Part model, mm, in its own coordinate system. Give positions to 0.01 mm unless a question says otherwise; leave off trailing zeros. Write each loop counter-clockwise with the first axis right and the second up, starting at its lowest first coordinate (ties: lowest second). Pieces come first, ordered by that corner, then holes. Notation, with made-up numbers: (42, -5.5) - (46, -5.5) arc R11 cw to (46, 7.5) - close; hole circle Ø5 at (-26.5, 58.5). An arc over 180 degrees is marked (long way). Answer in a Markdown table with one row per item. Add a question column.
1. Probe line 1 along X through (y, z) = (-2.5, -51.05); line 2 along Y through (x, z) = (-9.5, -51.05); line 3 along X through (y, z) = (1, -51.1). List the from-to ranges inside material, lowest first.
2. Band-saw the part on B-B on y = 9. Write the cut outline in (x, z), plus the area to 3 significant figures.
3. Band-saw the part on D-D on y = -2. Write the cut outline in (x, z), plus the area to 3 significant figures.
4. Band-saw the part on A-A on x = -17. Write the cut outline in (y, z).
5. Band-saw the part on C-C on x = -8.5. Write the cut outline in (y, z).
```python
from build123d import *

# Parameters (mm, degrees)
EXTRUDE_START       = -3.8
SKETCH_1_R          = 25.801076528
SKETCH_1_R_2        = 1.549997321
SKETCH_1_R_3        = 1.54999944
EXTRUDE_1_DEPTH     = 0.2
CUT_EXTRUDE_START   = -3.8
SKETCH_2_W          = 3.794
SKETCH_2_H          = 3.794
SKETCH_2_W_2        = 4.175
SKETCH_2_H_2        = 4.556
SKETCH_2_W_3        = 4.048
SKETCH_2_H_3        = 4.683
CUT_EXTRUDE_1_DEPTH = 0.2
CUT_EXTRUDE_2_DEPTH = 0.2
CUT_EXTRUDE_3_DEPTH = 0.2
CUT_EXTRUDE_4_DEPTH = 0.2
CUT_EXTRUDE_5_DEPTH = 0.2


with BuildPart() as part:
    # 草图1 → 凸台-拉伸1 (new body)
    with BuildSketch(Plane(origin=(0, 0, -54.8040151), x_dir=(-1, 0, 0), z_dir=(0, 0, -1)).offset(EXTRUDE_START)):
        with Locations(Location((24.698490112, -1.512152456, 0), (0, 0, 180))):
            Circle(SKETCH_1_R)
        with Locations(Location((24.698490112, 21.537847164, 0), (0, 0, 180))):
            Circle(SKETCH_1_R_2, mode=Mode.SUBTRACT)
        with Locations(Location((24.698490112, -24.562152076, 0), (0, 0, 180))):
            Circle(SKETCH_1_R_3, mode=Mode.SUBTRACT)
    extrude(amount=EXTRUDE_1_DEPTH)

    # 草图2 → 切除-拉伸1 (cut)
    with BuildSketch(Plane(origin=(0, 0, -54.8040151), x_dir=(-1, 0, 0), z_dir=(0, 0, -1)).offset(CUT_EXTRUDE_START)):
        with Locations((23.362494109, -1.270150744)):
            Rectangle(SKETCH_2_W, SKETCH_2_H)
        with Locations((34.093992827, 9.14385072)):
            Rectangle(SKETCH_2_W_2, SKETCH_2_H_2)
        with Locations((41.967993376, 9.397848523)):
            Rectangle(SKETCH_2_W_2, SKETCH_2_H_2)
        with Locations((34.157492278, -11.874650561)):
            Rectangle(SKETCH_2_W_3, SKETCH_2_H_3)
        with Locations((42.031492827, -11.874650561)):
            Rectangle(SKETCH_2_W_3, SKETCH_2_H_3)
    extrude(amount=CUT_EXTRUDE_1_DEPTH, mode=Mode.SUBTRACT)

    # 草图3 → 切除-拉伸2 (cut)
    with BuildSketch(Plane(origin=(0, 0, -54.8040151), x_dir=(-1, 0, 0), z_dir=(0, 0, -1)).offset(CUT_EXTRUDE_START)):
        Polygon((15.882224059, 13.556279819), (9.63139829, 7.305454051), (2.996403479, 13.940448863), (9.247230868, 20.191276253), align=None)
    extrude(amount=CUT_EXTRUDE_2_DEPTH, mode=Mode.SUBTRACT)

    # 草图4 → 切除-拉伸3 (cut)
    with BuildSketch(Plane(origin=(0, 0, -54.8040151), x_dir=(-1, 0, 0), z_dir=(0, 0, -1)).offset(CUT_EXTRUDE_START)):
        Polygon((7.030438471, 4.406785556), (7.030438471, 6.006785556), (10.230438471, 6.006785556), (10.230438471, 4.406785556), (8.630438471, 4.406785556), align=None)
        Polygon((7.030438471, 0.086785556), (7.030438471, 1.686785556), (10.230438471, 1.686785556), (10.230438471, 0.086785556), (8.630438471, 0.086785556), align=None)
        Polygon((7.030438471, -4.363214444), (7.030438471, -2.763214444), (10.230438471, -2.763214444), (10.230438471, -4.363214444), (8.630438471, -4.363214444), align=None)
        Polygon((7.030438471, -9.573214444), (7.030438471, -7.973214444), (10.230438471, -7.973214444), (10.230438471, -9.573214444), (8.630438471, -9.573214444), align=None)
    extrude(amount=CUT_EXTRUDE_3_DEPTH, mode=Mode.SUBTRACT)

    # 草图5 → 切除-拉伸4 (cut)
    with BuildSketch(Plane(origin=(0, 0, -54.8040151), x_dir=(-1, 0, 0), z_dir=(0, 0, -1)).offset(CUT_EXTRUDE_START)):
        Polygon((14.853491423, 2.675851453), (12.053491423, 2.675851453), (12.053491423, -5.724148547), (14.853491423, -5.724148547), (18.028494414, -5.724148547), (18.028494414, -3.124148547), (20.128494414, -3.124148547), (20.128494414, 0.075851453), (18.028494414, 0.075851453), (18.028494414, 2.675851453), (17.653491423, 2.675851453), align=None)
    extrude(amount=CUT_EXTRUDE_4_DEPTH, mode=Mode.SUBTRACT)

    # 草图7 → 切除-拉伸5 (cut)
    with BuildSketch(Plane(origin=(0, 0, -54.8040151), x_dir=(-1, 0, 0), z_dir=(0, 0, -1)).offset(CUT_EXTRUDE_START)):
        with BuildLine():
            Line((50.959593828, -3.679110402), (50.311348997, -3.679110402))
            Line((50.311348997, -3.679110402), (47.368920104, -3.679058566))
            ThreePointArc((47.368920104, -3.679058566), (46.803238807, -3.444734025), (46.568934198, -2.879044472))
            Line((46.568934198, -2.879044472), (46.568983525, -0.079044473))
            ThreePointArc((46.568983525, -0.079044473), (46.803308066, 0.486636824), (47.368997619, 0.720941434))
            Line((47.368997619, 0.720941434), (50.305693305, 0.720889698))
            Line((50.305693305, 0.720889698), (50.959593828, 0.720889698))
            Line((50.959593828, 0.720889698), (50.959593828, -3.679110402))
        make_face()
        with BuildLine():
            Line((-1.005097138, 0.720889698), (1.931598548, 0.720941434))
            ThreePointArc((1.931598548, 0.720941434), (2.497288101, 0.486636824), (2.731612641, -0.079044473))
            Line((2.731612641, -0.079044473), (2.731661969, -2.879044472))
            ThreePointArc((2.731661969, -2.879044472), (2.49735736, -3.444734025), (1.931676063, -3.679058566))
            Line((1.931676063, -3.679058566), (-1.01075283, -3.679110402))
            Line((-1.01075283, -3.679110402), (-1.658997661, -3.679110402))
            Line((-1.658997661, -3.679110402), (-1.658997661, 0.720889698))
            Line((-1.658997661, 0.720889698), (-1.005097138, 0.720889698))
        make_face()
    extrude(amount=CUT_EXTRUDE_5_DEPTH, mode=Mode.SUBTRACT)


solid = part.part
```
Values:
| question | item | result |
|---|---|---|
| 1 | line 1 | x = -46.57 to -25.26, -21.47 to -20.13, -12.05 to -2.73 |
| 1 | line 2 | y = -22.36 to -9.57, -7.97 to -4.36, -2.76 to 0.09, 1.69 to 4.41, 6.01 to 7.44 |
| 1 | line 3 | x = -50.38 to -18.03, -12.05 to -10.23, -7.03 to 0.98 |
| 2 | outline | (-48.26, -51.2) - (-44.06, -51.2) - (-44.06, -51) - (-48.26, -51) - close; (-39.88, -51.2) - (-36.18, -51.2) - (-36.18, -51) - (-39.88, -51) - close; (-32.01, -51.2) - (-11.33, -51.2) - (-11.33, -51) - (-32.01, -51) - close; (-7.94, -51.2) - (-1.14, -51.2) - (-1.14, -51) - (-7.94, -51) - close |
| 2 | area | 7.08 mm² |
| 3 | outline | (-46.57, -51.2) - (-25.26, -51.2) - (-25.26, -51) - (-46.57, -51) - close; (-21.47, -51.2) - (-20.13, -51.2) - (-20.13, -51) - (-21.47, -51) - close; (-12.05, -51.2) - (-2.73, -51.2) - (-2.73, -51) - (-12.05, -51) - close |
| 3 | area | 6.39 mm² |
| 4 | outline | (-26.14, -51.2) - (-5.72, -51.2) - (-5.72, -51) - (-26.14, -51) - close; (2.68, -51.2) - (23.11, -51.2) - (23.11, -51) - (2.68, -51) - close |
| 5 | outline | (-21.59, -51.2) - (-9.57, -51.2) - (-9.57, -51) - (-21.59, -51) - close; (-7.97, -51.2) - (-4.36, -51.2) - (-4.36, -51) - (-7.97, -51) - close; (-2.76, -51.2) - (0.09, -51.2) - (0.09, -51) - (-2.76, -51) - close; (1.69, -51.2) - (4.41, -51.2) - (4.41, -51) - (1.69, -51) - close; (6.01, -51.2) - (8.44, -51.2) - (8.44, -51) - (6.01, -51) - close |
